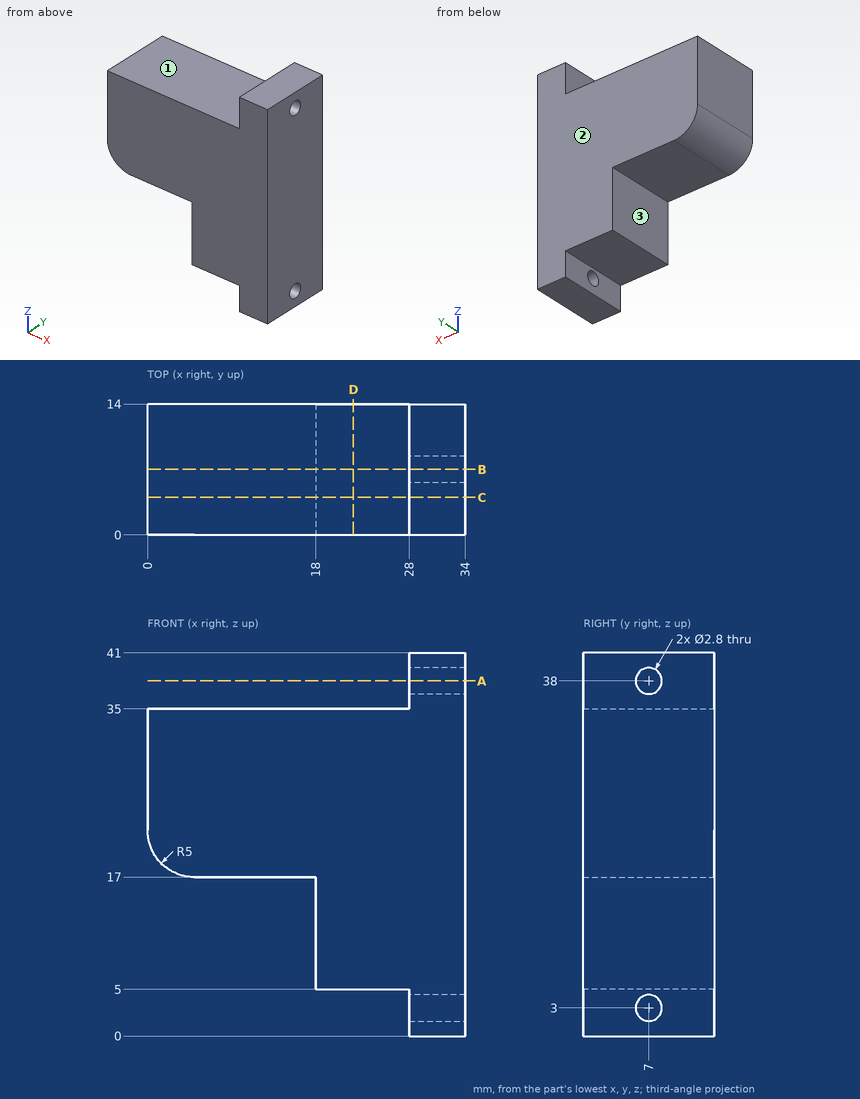
Drawing for the job (mm, zero at the part's lowest x, y, z). A direction names the side the tool comes from. Give positions to 0.01 mm unless a question says otherwise; leave off trailing zeros. Order: outer loops, then holes, each group sorted by start corner. A loop starts at its lowest first (then second) coordinate and runs counter-clockwise, first axis right, second up. Notation, with made-up numbers: (-20.5, -27.75) -> (-7.5, -27.75) arc R31 ccw to (-7.5, 9.25) -> close; hole circle Ø10 at (76.5, 54). An arc over 180 degrees is marked (long way). Use one line per item in the form item = value.
(1) Saw through at C-C (y = 4). Write the cut outline in (x, z), then the cut area to 3 significant figures.
Solution:
outline = (0, 22) arc R5 ccw to (5, 17) -> (18, 17) -> (18, 5) -> (28, 5) -> (28, 0) -> (34, 0) -> (34, 41) -> (28, 41) -> (28, 35) -> (0, 35) -> close
area = 865 mm²
(2) Saw through at D-D (x = 22). Write the cut outline in (y, z).
Solution:
outline = (0, 5) -> (14, 5) -> (14, 35) -> (0, 35) -> close
(3) Saw through at A-A (z = 38). Write the cut outline in (x, y), then the cut area to 3 significant figures.
Solution:
outline = (28, 0) -> (34, 0) -> (34, 5.6) -> (28, 5.6) -> close; (28, 8.4) -> (34, 8.4) -> (34, 14) -> (28, 14) -> close
area = 67.2 mm²
(4) Drill centre lines: line 1 (Y direction, x = 30.1, z = 38); line 2 (Z direction, x = 25, y = 4.5); line 3 (X direction, y = 5.5, z = 3). Where is each one in solid material? Low to high. Write a range as from..to.
Solution:
line_1 = 0..5.6, 8.4..14
line_2 = 5..35
line_3 = 28..34
(5) Flat gauge pins, fed straight in: P1, Ø4, axis at x = 23.5, y = 9, coming from the -Z side; P2, Ø2.5, axis at y = 7, z = 38, coming from the -X side; P3, Ø8, axis at y = 5.5, z = 17.5, coming from the -X side; P4, Ø1.8, axis at y = 5, z = 37.5, coming from the -X side. Where does each tip first touch, or does it go through?
Solution:
P1 = 5
P2 = through
P3 = 0.03
P4 = 28
(6) Saw through at B-B (y = 7). Write the cut outline in (x, z).
Solution:
outline = (0, 22) arc R5 ccw to (5, 17) -> (18, 17) -> (18, 5) -> (28, 5) -> (28, 4.4) -> (34, 4.4) -> (34, 36.6) -> (28, 36.6) -> (28, 35) -> (0, 35) -> close; (28, 0) -> (34, 0) -> (34, 1.6) -> (28, 1.6) -> close; (28, 39.4) -> (34, 39.4) -> (34, 41) -> (28, 41) -> close
(7) Tool access for the marked faces 1, 2 and 3: list every direction of +Z, -Z, +X, -X, +Y, -Y with a clear straight run to the whole face (end or side of a thin tool).
Solution:
face_1 = +Z, -X, +Y, -Y
face_2 = +Z, -Z, +X, -X, +Y
face_3 = -Z, -X, +Y, -Y
